from build123d import *

# Parameters (mm, degrees)
SKETCH1_R     = 49.53
BODY_DEPTH    = 9.525
SKETCH2_R     = 42.426526601
SKETCH2_R_2   = 36.076526601
FLANGE_DEPTH  = 8.255
FILLET1_R     = 5.08
CHAMFER1_SIZE = 0.508


with BuildPart() as part:
    # Sketch1 → body (new body)
    with BuildSketch(Plane(origin=(0, 0, 0), x_dir=(1, 0, 0), z_dir=(0, 1, 0))):
        with Locations(Location((0, 0, 0), (0, 0, 90))):
            Circle(SKETCH1_R)
    extrude(amount=BODY_DEPTH)

    # Sketch2 → flange (add)
    with BuildSketch(Plane.XZ):
        with Locations(Location((0, 0, 0), (0, 0, 90))):
            Circle(SKETCH2_R)
        with Locations(Location((0, 0, 0), (0, 0, 270))):
            Circle(SKETCH2_R_2, mode=Mode.SUBTRACT)
    extrude(amount=FLANGE_DEPTH)

    # Fillet1
    fillet1_edges = [part.edges().sort_by_distance(p)[0] for p in [
        (0, 9.525, 49.53),
    ]]
    fillet(fillet1_edges, radius=FILLET1_R)

    # Chamfer1
    chamfer1_edges = [part.edges().sort_by_distance(p)[0] for p in [
        (0, -8.255, -42.426526601),
        (0, -8.255, 36.076526601),
    ]]
    chamfer(chamfer1_edges, length=CHAMFER1_SIZE)


solid = part.part
Design review of the part built by this model. Coordinates are the model's own, in mm. A direction names the side the tool comes from. Coordinates: 2 decimals unless noted, no trailing zeros. Write each loop counter-clockwise with the first axis right and the second up, starting at its lowest first coordinate (ties: lowest second). Pieces come first, ordered by that corner, then holes. Notation, with made-up numbers: (-27, 30) -> (5, 30) arc R27 ccw to (5, 59) -> close; hole circle Ø11 at (-21.75, 9). An arc over 180 degrees is marked (long way). Write each question's results on one line, items separated by ' | '. Start each with the question number.
(1) Tool access review of faces 4 (the face through (-22.2, 0, -36.5)), 5 (the face through (-37, -8.255, 3)): name each direction out of +Z, -Z, +X, -X, +Y, -Y from which nothing blocks a thin tool from reaching the whole face with its end or side.
(2) Take a section at A-A on x = 0. Write out the cut boundary in (y, z) (3 decimals), and give its area (3 significant figures).
(3) Take a section at C-C on y = -2.5. Write out the cut boundary in (x, z), and give its area (3 significant figures).
(4) Clearance check with flat-ended pins moving along their axes: P1, Ø10, axis at x = -16.5, z = -18.5, coming from the -Y side; P2, Ø4, axis at x = 14.5, y = -1.5, coming from the +Z side (3 decimals); P3, Ø1, axis at y = 4.5, z = -3.5, coming from the +X side. State where each tip first meets the part, or that it passes through.
(5) The part is to be moulded in two halves that separate along X. For faces 1 (the face through (-1, 9.525, 1)), 2 (the face through (10.84, -3.82, -34.41)), 3 (the face through (-14.88, 2.19, -47.24)), say which applies: pulls with the +X half, pulls with the -X half, needs draft (parallel to the pull), parting line crosses it, or undercut.
(6) Take a section at B-B on z = 0. Write out the cut boundary in (x, y) (3 decimals), and give its area (3 significant figures).
(7) For line 1 along X through (y, z) = (-5.25, 0); line 2 along Y through (x, z) = (-11.5, -8) (3 decimals); line 3 along Z through (x, y) = (30, -1.25), list the stretches that pass through material, from the lowest coordinate up. Write a range as from..to.
Results found:
1) face 4: -Y | face 5: +Z, -Z, +X, -X, -Y
2) outline: (-8.255, -41.919) -> (-7.747, -42.427) -> (0, -42.427) -> (0, -49.53) -> (4.445, -49.53) arc R5.08 ccw to (9.525, -44.45) -> (9.525, 44.45) arc R5.08 ccw to (4.445, 49.53) -> (0, 49.53) -> (0, 42.427) -> (-7.747, 42.427) -> (-8.255, 41.919) -> (-8.255, 36.585) -> (-7.747, 36.077) -> (0, 36.077) -> (0, -36.077) -> (-7.747, -36.077) -> (-8.255, -36.585) -> close | area: 1,040 mm2
3) outline: circle Ø84.85 at (0, 0); hole circle Ø72.15 at (0, 0) | area: 1,570 mm2
4) P1: stops at y = 0 | P2: stops at z = 47.745 | P3: stops at x = 49.44
5) face 1: needs draft | face 2: undercut | face 3: parting line crosses it
6) outline: (-49.53, 0) -> (-42.427, 0) -> (-42.427, -7.747) -> (-41.919, -8.255) -> (-36.585, -8.255) -> (-36.077, -7.747) -> (-36.077, 0) -> (36.077, 0) -> (36.077, -7.747) -> (36.585, -8.255) -> (41.919, -8.255) -> (42.427, -7.747) -> (42.427, 0) -> (49.53, 0) -> (49.53, 4.445) arc R5.08 ccw to (44.45, 9.525) -> (-44.45, 9.525) arc R5.08 ccw to (-49.53, 4.445) -> close | area: 1,040 mm2
7) line 1: x = -42.43..-36.08, 36.08..42.43 | line 2: y = 0..9.525 | line 3: z = -30..-20.04, 20.04..30
